Check sheet for the modelled part. Datum: model origin and axes. Units: mm. A direction names the side the tool comes from. Round coordinates to 2 decimals unless told otherwise and drop trailing zeros. Order: outer loops, then holes, each group sorted by start corner. A loop starts at its lowest first (then second) coordinate and runs counter-clockwise, first axis right, second up. Notation, with made-up numbers: (31, 45) -> (42, 45) arc R29 cw to (42, 65) -> close; hole circle Ø1 at (-31, 55.5). An arc over 180 degrees is marked (long way). Answer in a Markdown table with one row per item. Add a question column.
1. Sectioned sample at D-D, the plane y = -24. Record the boundary of the cut face in (x, z).
2. Depth check by flat-ended pin: P1, Ø3, axis at y = -10.16, z = 9.525, coming from the -X side; P2, Ø5, axis at x = 3, z = 115.5, coming from the +Y side; P3, Ø14, axis at y = -7, z = 89.5, coming from the -X side; P4, Ø3, axis at x = 2, z = 135, coming from the -Y side. Enter the tip coordinate at first touch or a pass-through.
3. Material ranges on L1, parallel to Z at x = 11, y = -10.16; L2, parallel to X at y = -6.5, z = 228; L3, parallel to Y at x = 3.25, z = 26.5, recorded low to high. Write a range as from..to.
4. Access from +Z, -Z, +X, -X, +Y, -Y to the whole of each face (thin tool, end or side, straight path). Record for faces 1 (the flat face through (3, -16.51, 126)), 2 (the cylindrical face through (9.481, -7.895, 8.347)).
5. Draft check along Z on faces 3 (the flat face through (3, -3.81, 126)), 4 (the flat face through (8, -10, 247.65)), 5 (the cylindrical face through (9.481, -10.272, 69.225)). Enter one of: +Z half, -Z half, draft (parallel to the pull), parting line (faces both ways), or undercut.
6. Sectioned sample at A-A, the plane x = 3. Record the boundary of the cut face in (y, z).
7. Sectioned sample at C-C, the plane z = 100.5. Record the boundary of the cut face in (x, y).
8. Sectioned sample at B-B, the plane y = -10.16. Record the boundary of the cut face in (x, z).
Autodesk Inventor part; units mm, degrees
ref_plane "Work Plane1" through (6.35, -20.32, 0) normal (1, 0, 0) x (0, 0, -1)
ref_plane "Work Plane2" through (0, -10.16, 0) normal (0, 1, 0) x (-1, 0, 0)
ref_plane "YZ Plane" through (0, 0, 0) normal (1, 0, 0) x (0, 1, 0)
sketch "Sketch1" plane through (0, 0, 0) normal (0, 0, 1) x (1, 0, 0)
  line L0 (0, 0) -> (12.7, 0)
  line L1 (12.7, 0) -> (12.7, -20.32)
  line L2 (12.7, -20.32) -> (0, -20.32)
  line L3 (0, -20.32) -> (0, 0)
  line L4 (0, 0) -> (6.35, 6.35)
  line L5 (12.7, -20.32) -> (6.35, -26.67)
  line L6 (6.35, -26.67) -> (0, -20.32)
  line L7 (6.35, 6.35) -> (12.7, 0)
  dimension "d0" = 90
  dimension "d1" = 90
  dimension "d2" = 33.02
  dimension "d3" = 12.7
extrude "Extrusion1" add sketch "Sketch1" along normal blind 247.65
sketch "Sketch6" plane through (0, 0, 247.65) normal (0, 0, 1) x (1, 0, 0)
  line L0 (-5.8804, -3.81) -> (6.35, -3.81)
  line L1 (6.35, -3.81) -> (6.35, -16.51)
  line L2 (6.35, -16.51) -> (-5.8804, -16.51)
  line L3 (-5.8804, -16.51) -> (-5.8804, -3.81)
  line L4 (12.7, -20.32) -> (12.7, 0)
  line L5 (0, 0) -> (0, -20.32)
  point P0 (6.35, -10.16)
  point P1 (12.7, -10.16)
  dimension "d43" = 12.7
  dimension "d44" = 6.35
extrude "Extrusion5" cut sketch "Sketch6" against normal through all
ref_plane "Work Plane1" through (6.35, -20.32, 0) normal (1, 0, 0) x (0, 0, -1)
ref_plane "Work Plane2" through (0, -10.16, 0) normal (0, 1, 0) x (-1, 0, 0)
sketch "Sketch2" plane through (12.7, -20.32, 0) normal (1, 0, 0) x (0, 0, -1)
  line L0 (-247.65, 0) -> (-247.65, 20.32)
  line L1 (0, 20.32) -> (-247.65, 20.32)
  line L2 (0, 20.32) -> (0, 0)
  line L3 (0, 0) -> (-247.65, 0)
  circle A0 centre (-238.125, 10.16) radius 4.7625
  circle A1 centre (-9.525, 10.16) radius 4.7625
  line L4 (-233.3625, 16.7388) -> (-233.3625, 5.4122)
  line L5 (-14.2875, 15.6909) -> (-14.2875, 3.5669)
  point P0 (0, 10.16)
  point P1 (-180.975, 10.16)
  point P2 (-66.675, 10.16)
  point P3 (-123.825, 10.16)
  dimension "d28" = 9.525
  dimension "d47" = 9.525
  dimension "d48" = 57.15
  dimension "d49" = 57.15
  dimension "d51" = 9.525
  dimension "d52" = 219.075
  dimension "d56" = 57.15
  dimension "d59" = 228.6
  dimension "d60" = 57.15
hole "Hole2" at (12.7, -10.16, 9.525) at (12.7, -10.16, 180.975) at (12.7, -10.16, 66.675) at (12.7, -10.16, 238.125) at (12.7, -10.16, 123.825) direction (-1, 0, 0) diameter 5.1054 end through all
properties part number "SC Path" material "Aluminum 6061"
Answer key:
| question | item | result |
|---|---|---|
| 1 | outline | (3.68, 0) -> (9.02, 0) -> (9.02, 247.65) -> (3.68, 247.65) -> close |
| 2 | P1 | passes through |
| 2 | P2 | stops at y = 5.5 |
| 2 | P3 | stops at x = 0 |
| 2 | P4 | stops at y = -23.82 |
| 3 | L1 | z = 0..6.97, 12.08..64.12, 69.23..121.27, 126.38..178.42, 183.53..235.57, 240.68..247.65 |
| 3 | L2 | x = 6.35..12.7 |
| 3 | L3 | y = -23.57..-16.51, -3.81..3.25 |
| 4 | face 1 | +Z, -Z, -X |
| 4 | face 2 | +X, -X |
| 5 | face 3 | draft |
| 5 | face 4 | +Z half |
| 5 | face 5 | undercut |
| 6 | outline | (-23.32, 0) -> (-16.51, 0) -> (-16.51, 247.65) -> (-23.32, 247.65) -> close; (-3.81, 0) -> (3, 0) -> (3, 247.65) -> (-3.81, 247.65) -> close |
| 7 | outline | (0, -20.32) -> (6.35, -26.67) -> (12.7, -20.32) -> (12.7, 0) -> (6.35, 6.35) -> (0, 0) -> (0, -3.81) -> (6.35, -3.81) -> (6.35, -16.51) -> (0, -16.51) -> close |
| 8 | outline | (6.35, 0) -> (12.7, 0) -> (12.7, 6.97) -> (6.35, 6.97) -> close; (6.35, 12.08) -> (12.7, 12.08) -> (12.7, 64.12) -> (6.35, 64.12) -> close; (6.35, 69.23) -> (12.7, 69.23) -> (12.7, 121.27) -> (6.35, 121.27) -> close; (6.35, 126.38) -> (12.7, 126.38) -> (12.7, 178.42) -> (6.35, 178.42) -> close; (6.35, 183.53) -> (12.7, 183.53) -> (12.7, 235.57) -> (6.35, 235.57) -> close; (6.35, 240.68) -> (12.7, 240.68) -> (12.7, 247.65) -> (6.35, 247.65) -> close |
